CAD build for the part. Positions are in the model's coordinates, mm. A direction names the side the tool comes from. Give positions to 0.01 mm unless a question says otherwise; leave off trailing zeros. Loops run counter-clockwise (first coordinate to the right, second up) from the corner with the lowest first, then second, coordinate; pieces in that order, holes last. Notation, with made-up numbers: (33, 8.5) -> (92, 8.5) arc R5 cw to (92, 12.5) -> close; hole circle Ø1 at (71.5, 59). An arc over 180 degrees is marked (long way). Use one line per item in the form item = value.
```python
from build123d import *

# Parameters (mm, degrees)
F3_DEPTH = 3.175


with BuildPart() as f1:
    # F0 (on Front) → F1 (revolve)
    with BuildSketch(Plane.XZ):
        with BuildLine():
            Line((0, 0), (0, 50.8))
            Line((0, 50.8), (0, 53.3654))
            ThreePointArc((0, 53.3654), (-2.626821, 52.680442), (-4.5847, 50.8))
            Line((-4.5847, 50.8), (-2.413, 50.8))
            Line((-2.413, 50.8), (-2.413, 0))
            Line((-2.413, 0), (0, 0))
        make_face()
    revolve(axis=Axis((0, 0, 25.4), (0, 0, -1)))

    # F2 (on face) → F3 (join)
    with BuildSketch(Plane(origin=(0, 0, 0), x_dir=(1, 0, 0), z_dir=(0, 0, -1))):
        Polygon((2.749631, 4.7625), (-2.749631, 4.7625), (-5.499261, 0), (-2.749631, -4.7625), (2.749631, -4.7625), (5.499261, 0), align=None)
    extrude(amount=F3_DEPTH)


solid = f1.part
```
1. Mould opens along Z. For faces 3 (the flat face through (0, 0, -3.175)), 4 (the flat face through (-2, -2, 50.8)), 5 (the flat face through (2.4, -1.1, 0)), 6 (the flat face through (0, -4.762, -2)) say: pulls with the +Z half, pulls with the -Z half, needs draft (parallel to the pull), parting line crosses it, or undercut.
Result sheet:
face_3 = pulls with the -Z half
face_4 = undercut
face_5 = undercut
face_6 = needs draft
2. Tool access for faces 1 (the flat face through (4.11, 2.41, -1.57)), 2 (the cylindrical face through (1.915, -1.468, 25.044)): list every direction of +Z, -Z, +X, -X, +Y, -Y with a clear straight run to the whole face (end or side of a thin tool).
Result sheet:
face_1 = +Z, -Z, +X, +Y
face_2 = none
3. Drill centre lines: line 1 (Z direction, x = -3.25, y = -2.5) (3 decimals); line 2 (Z direction, x = 2.75, y = -3.5) (3 decimals); line 3 (X direction, y = 0.75, z = 20.5). Where is each one in solid material? Low to high.
Result sheet:
line_1 = -3.175 to 0, 50.8 to 51.468
line_2 = -3.175 to 0, 50.8 to 51.007
line_3 = -2.29 to 2.29
4. Cut at A-A, the plane z = 45. Write the cut outline in (x, y), then the cut area to 3 significant figures.
Result sheet:
outline = circle Ø4.83 at (0, 0)
area = 18.3 mm^2
5. Drop flat-ended pins along their axis: P1, Ø6, axis at x = -4, z = 26.5, coming from the -Y side; P2, Ø5, axis at x = 4, z = 31, coming from the +Y side; P3, Ø1, axis at x = 0.5, y = -2.5, coming from the +Z side. Give the stop position or say it passes through.
Result sheet:
P1 = -2.2
P2 = 1.89
P3 = 52.96
